The model under review builds one solid part; all positions refer to its coordinate system, in mm. Face numbers are marked on the shaded views. Round coordinates to 2 decimals unless told otherwise and drop trailing zeros. Order: outer loops, then holes, each group sorted by start corner. A loop starts at its lowest first (then second) coordinate and runs counter-clockwise, first axis right, second up. Notation, with made-up numbers: M 0.5,27 L 7.5,27 A28 ccw 7.5,53 Z; hole C 4,58 d1. An arc over 180 degrees is marked long. One line per item, written item: value. Start each with the question number.
from build123d import *

# Parameters (mm, degrees)
SKETCH1_R           = 3.96875
SKETCH1_R_2         = 1.905
BOSS_EXTRUDE1_DEPTH = 12.7
FILLET1_R           = 2.54


with BuildPart() as part:
    # Sketch1 → Boss-Extrude1 (new body)
    with BuildSketch(Plane.XY):
        with BuildLine():
            Line((-6.35, -31.75), (-6.35, 6.35))
            Line((-6.35, 6.35), (-13.877185568, 49.038790666))
            Line((-13.877185568, 49.038790666), (-45.239836887, 43.508709052))
            Line((-45.239836887, 43.508709052), (-34.93811028, 58.221099372))
            Line((-34.93811028, 58.221099372), (-3.765469283, 63.71767704))
            Line((-3.765469283, 63.71767704), (6.35, 6.35))
            Line((6.35, 6.35), (6.35, -31.75))
            ThreePointArc((6.35, -31.75), (0, -38.1), (-6.35, -31.75))
        make_face()
        Circle(SKETCH1_R, mode=Mode.SUBTRACT)
        with Locations((0, -31.75)):
            Circle(SKETCH1_R_2, mode=Mode.SUBTRACT)
    extrude(amount=BOSS_EXTRUDE1_DEPTH)

    # Fillet1
    fillet1_edges = [part.edges().sort_by_distance(p)[0] for p in [
        (-6.35, 6.35, 6.35),
        (-13.877185568, 49.038790666, 6.35),
        (-45.239836887, 43.508709052, 6.35),
        (-34.93811028, 58.221099372, 6.35),
        (-3.765469283, 63.71767704, 6.35),
        (6.35, 6.35, 6.35),
    ]]
    fillet(fillet1_edges, radius=FILLET1_R)


solid = part.part
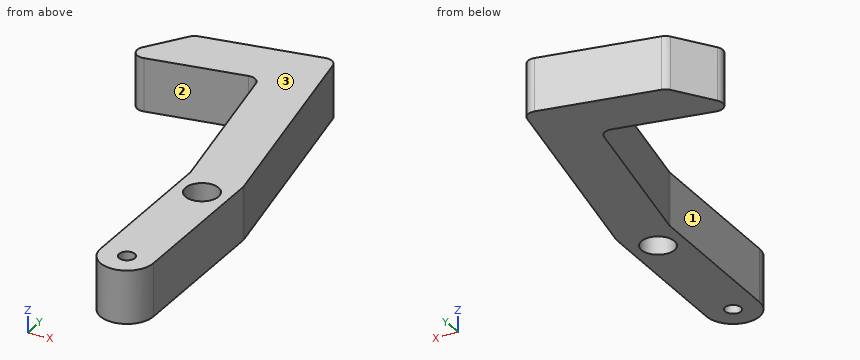
Item 1: Consider section B-B, the plane y = 0. Give the boundary of the cut face in (x, z).
Item 2: Wall thickness on L1, parallel to X at y = -5.5, z = 9.75; L2, parallel to X at y = -33, z = 11.75; L3, parallel to X at y = -30, z = 6.25: over which ranges is each line inside the solid? List them lowest first.
Item 3: Consider section C-C, the plane x = 0. Give the boundary of the cut face in (y, z) (3 decimals), then the cut area to 3 significant figures.
Item 4: Consider section D-D, the plane y = 30.5. Give the boundary of the cut face in (x, z).
Item 5: Consider section A-A, the plane z = 1.25. Count the separate pieces of the cut face and the enclosed holes in it, then the cut area to 3 significant figures.
Item 6: The part is to be moulded in two halves that separate along X. For the marked faces 1, 2 and 3, say which applies: pulls with the +X half, pulls with the -X half, needs draft (parallel to the pull), parting line crosses it, or undercut.
Item 7: Clearance check with flat-ended pins moving along their axes: P1, Ø4, axis at y = -20.5, z = 8, coming from the -X side; P2, Ø1.5, axis at y = 12.5, z = 5, coming from the +X side; P3, Ø3.5, axis at x = 0, y = -31.75, coming from the -Z side; P4, Ø1.5, axis at x = -27, z = 5, coming from the +Y side. State where each tip first meets the part, or that it passes through.
Computed:
1. outline: M -6.35,0 L -3.97,0 L -3.97,12.7 L -6.35,12.7 Z; M 3.97,0 L 6.35,0 L 6.35,12.7 L 3.97,12.7 Z
2. L1: x = -6.35 to 6.35
2. L2: x = -6.23 to -1.44, 1.44 to 6.23
2. L3: x = -6.35 to -0.75, 0.75 to 6.35
3. outline: M -38.1,0 L -33.655,0 L -33.655,12.7 L -38.1,12.7 Z; M -29.845,0 L -3.969,0 L -3.969,12.7 L -29.845,12.7 Z; M 3.969,0 L 42.363,0 L 42.363,12.7 L 3.969,12.7 Z
3. area: 873 mm^2
4. outline: M -10.61,0 L 2.09,0 L 2.09,12.7 L -10.61,12.7 Z
5. separate pieces: 1
5. enclosed holes: 2
5. area: 1,520 mm^2
6. face 1: pulls with the -X half
6. face 2: undercut
6. face 3: needs draft
7. P1: stops at x = -6.35
7. P2: stops at x = 5.4
7. P3: passes through
7. P4: stops at y = 59.75
